Here's the drawing with two shaded views (mm, measured from the low corner). I have some questions. A direction names the side the tool comes from. Round coordinates to 2 decimals unless told otherwise and drop trailing zeros. Loops run counter-clockwise (first coordinate to the right, second up) from the corner with the lowest first, then second, coordinate; pieces in that order, holes last.
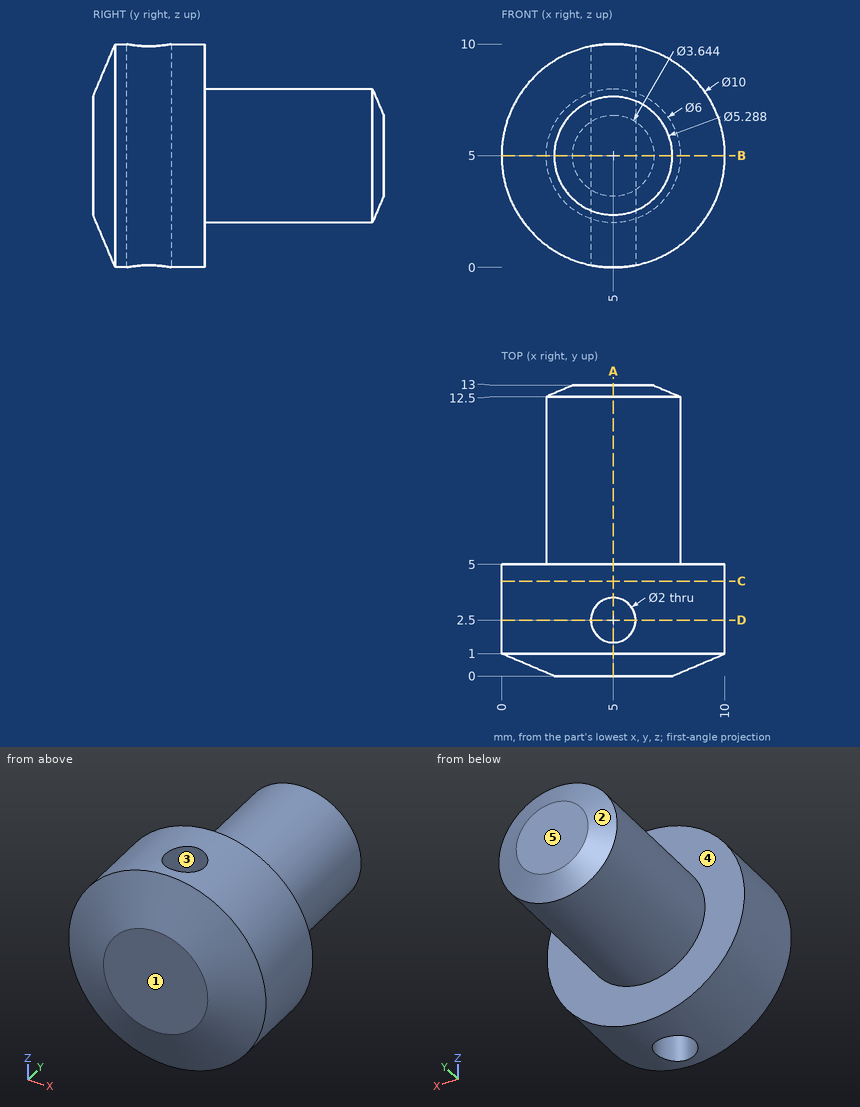
Item 1: If we section it at A-A, the plane x = 5: Please give me the cut outline in (y, z).
Results list:
outline: (0, 2.36) - (1, 0) - (1.5, 0) - (1.5, 10) - (1, 10) - (0, 7.64) - close; (3.5, 0) - (5, 0) - (5, 2) - (12.5, 2) - (13, 3.18) - (13, 6.82) - (12.5, 8) - (5, 8) - (5, 10) - (3.5, 10) - close
Item 2: For the marked faces 4 and 5, which set-ups out of +Z, -Z, +X, -X, +Y, -Y let a thin tool reach every point of the face, with its end or its side?
Results list:
face 4: +Y
face 5: +Z, -Z, +X, -X, +Y
Item 3: We'd pull the mould along X, two halves only. Please class the marked faces 1, 2 and 3: released by +X, released by -X, zero draft, split by the parting line, or undercut.
Results list:
face 1: zero draft
face 2: split by the parting line
face 3: undercut
Item 4: If we section it at B-B, the plane z = 5: Please give me the cut outline in (x, y).
Results list:
outline: (0, 1) - (2.36, 0) - (7.64, 0) - (10, 1) - (10, 5) - (8, 5) - (8, 12.5) - (6.82, 13) - (3.18, 13) - (2, 12.5) - (2, 5) - (0, 5) - close; hole circle Ø2 at (5, 2.5)
Item 5: If we section it at C-C, the plane y = 4.25: Please give me the cut outline in (x, z).
Results list:
outline: circle Ø10 at (5, 5)
Item 6: Will these pins go through, and if not, where does the flat tip stop? pin 1 (1 mm diameter, centred on y = 9.5, z = 6.5, fed in from +X); pin 2 (1 mm diameter, centred on x = 2, y = 10.5, fed in from +Z); pin 3 (1.5 mm diameter, centred on x = 8.5, z = 4.5, fed in from -Y).
Results list:
pin 1: stops at x = 7.83
pin 2: stops at z = 6.66
pin 3: stops at y = 0.06
Item 7: If I drill on line 1 along X through (y, z) = (2.5, 3.75); line 2 along Y through (x, z) = (4.25, 9.5) (1 decimal); line 3 along X through (y, z) = (2.5, 3), over which ranges is the centre line in solid material (lowest first)?
Results list:
line 1: x = 0.16 to 4, 6 to 9.84
line 2: y = 0.8 to 1.8, 3.2 to 5
line 3: x = 0.42 to 4, 6 to 9.58
Item 8: If we section it at D-D, the plane y = 2.5: Please give me the cut outline in (x, z).
Results list:
outline: (4, 0.1) - (4, 9.9) arc R5 ccw to start; (6, 0.1) arc R5 ccw to (6, 9.9) - close
